For this review, take the finished solid that the model builds, in its own axes (mm). A direction names the side the tool comes from. Give positions to 0.01 mm unless a question says otherwise; leave off trailing zeros. Write each loop counter-clockwise with the first axis right and the second up, starting at its lowest first coordinate (ties: lowest second). Pieces come first, ordered by that corner, then holes. Notation, with made-up numbers: (87.5, 9) -> (117.5, 9) arc R14 ccw to (117.5, 32) -> close; hole circle Ø11 at (71, -5.75). An arc over 180 degrees is marked (long way). Write item = value, one per line.
```python
from build123d import *

# Parameters (mm, degrees)
SKETCH_1_R      = 1
EXTRUDE_1_DEPTH = 1.6
SKETCH_2_W      = 3
SKETCH_2_H      = 5
EXTRUDE_2_DEPTH = 1.47
SKETCH_3_W      = 8.226
SKETCH_3_H      = 4.069
EXTRUDE_3_DEPTH = 4.35


with BuildPart() as part:
    # 草图1 → 凸台-拉伸1 (new body)
    with BuildSketch(Plane.XY):
        with BuildLine():
            ThreePointArc((-10.538461538, -3.152907928), (0, -11), (10.538461538, -3.152907928))
            ThreePointArc((10.538461538, -3.152907928), (10.98391758, -2.370710612), (11.727272727, -1.863081957))
            ThreePointArc((11.727272727, -1.863081957), (13, 0), (11.727272727, 1.863081957))
            ThreePointArc((11.727272727, 1.863081957), (10.98391758, 2.370710612), (10.538461538, 3.152907928))
            ThreePointArc((10.538461538, 3.152907928), (0, 11), (-10.538461538, 3.152907928))
            ThreePointArc((-10.538461538, 3.152907928), (-10.98391758, 2.370710612), (-11.727272727, 1.863081957))
            ThreePointArc((-11.727272727, 1.863081957), (-13, 0), (-11.727272727, -1.863081957))
            ThreePointArc((-11.727272727, -1.863081957), (-10.98391758, -2.370710612), (-10.538461538, -3.152907928))
        make_face()
        with Locations((-11, 0)):
            Circle(SKETCH_1_R, mode=Mode.SUBTRACT)
        with Locations((11, 0)):
            Circle(SKETCH_1_R, mode=Mode.SUBTRACT)
    extrude(amount=EXTRUDE_1_DEPTH)

    # 草图2 → 凸台-拉伸2 (add)
    with BuildSketch(Plane.XY.offset(1.6)):
        Rectangle(SKETCH_2_W, SKETCH_2_H)
    extrude(amount=EXTRUDE_2_DEPTH)

    # 草图3 → 凸台-拉伸3 (add)
    with BuildSketch(Plane(origin=(0, 0, 0), x_dir=(-1, 0, 0), z_dir=(0, 0, -1))):
        with Locations((0, 7.8445)):
            Rectangle(SKETCH_3_W, SKETCH_3_H)
    extrude(amount=EXTRUDE_3_DEPTH)


solid = part.part
```
(1) Tool access review of faces 4 (the face through (0, 2.5, 2)), 5 (the face through (-1.5, 0, 2)), 6 (the face through (0, 5.81, -2)): name each direction out of +Z, -Z, +X, -X, +Y, -Y from which nothing blocks a thin tool from reaching the whole face with its end or side.
Answers below:
face_4 = +Z, +X, -X, +Y
face_5 = +Z, -X, +Y, -Y
face_6 = -Z, +X, -X, -Y
(2) Take a section at A-A (y = 0). Write out the cut boundary in (x, z), plus the area to 3 significant figures.
Answers below:
outline = (-13, 0) -> (-12, 0) -> (-12, 1.6) -> (-13, 1.6) -> close; (-10, 0) -> (10, 0) -> (10, 1.6) -> (1.5, 1.6) -> (1.5, 3.07) -> (-1.5, 3.07) -> (-1.5, 1.6) -> (-10, 1.6) -> close; (12, 0) -> (13, 0) -> (13, 1.6) -> (12, 1.6) -> close
area = 39.6 mm^2
(3) Take a section at B-B (z = 1). Write out the cut boundary in (x, y).
Answers below:
outline = (-11.73, -1.86) arc R2 cw to (-10.54, -3.15) arc R11 ccw to (10.54, -3.15) arc R2 cw to (11.73, -1.86) arc R2 ccw to (11.73, 1.86) arc R2 cw to (10.54, 3.15) arc R11 ccw to (-10.54, 3.15) arc R2 cw to (-11.73, 1.86) arc R2 ccw to start; hole circle Ø2 at (-11, 0); hole circle Ø2 at (11, 0)
(4) For pin 1 (1.6 mm diameter, centred on x = 0, z = 2.5, fed in from +Y); pin 2 (1.3 mm diameter, centred on x = -0.5, z = -1.5, fed in from +Y); pin 3 (2 mm diameter, centred on x = -2, z = -1.5, fed in from -Y), all flat-tipped, find the tip position at first contact; note any pin that passes through.
Answers below:
pin_1 = 2.5
pin_2 = 9.88
pin_3 = 5.81
(5) The part is to be moulded in two halves that separate along X. For faces 1 (the face through (1.5, 0, 2)), 2 (the face through (0, -11, 1)), 3 (the face through (-11.8, -0.6, 0.8)), say which applies: released by +X, released by -X, zero draft, split by the parting line, or undercut.
Answers below:
face_1 = released by +X
face_2 = split by the parting line
face_3 = undercut
(6) To check wall thickness, follow probe 1 along Z at (x, y) = (7, 5.5); probe 2 along Z at (x, y) = (3, 7.5); probe 3 along Y at (x, z) = (11, 0.5). State the ranges of each line that lie inside material, in increasing order.
Answers below:
probe_1 = 0 to 1.6
probe_2 = -4.35 to 1.6
probe_3 = -2.35 to -1, 1 to 2.35
(7) Take a section at D-D (z = -2.25). Write out the cut boundary in (x, y), plus the area to 3 significant figures.
Answers below:
outline = (-4.11, 5.81) -> (4.11, 5.81) -> (4.11, 9.88) -> (-4.11, 9.88) -> close
area = 33.5 mm^2
(8) Take a section at C-C (x = -11). Write out the cut boundary in (y, z), plus the area to 3 significant figures.
Answers below:
outline = (-2.35, 0) -> (-1, 0) -> (-1, 1.6) -> (-2.35, 1.6) -> close; (1, 0) -> (2.35, 0) -> (2.35, 1.6) -> (1, 1.6) -> close
area = 4.33 mm^2
